Read the model definition and answer for the solid it produces. Units are mm, in the model's axes. A direction names the side the tool comes from. Coordinates: 2 decimals unless noted, no trailing zeros. Write each loop counter-clockwise with the first axis right and the second up, starting at its lowest first coordinate (ties: lowest second). Pieces come first, ordered by that corner, then holes. Notation, with made-up numbers: (24, 15) -> (60, 15) arc R27 cw to (60, 36) -> close; hole circle Ø1 at (47, 2.5). An arc over 180 degrees is marked (long way). Return JSON: item names as keys, results as strings.
from build123d import *

# Parameters (mm, degrees)
SKETCH1_W           = 60.325
SKETCH1_H           = 21.59
REVOLVE2_ANGLE      = 19
CIRPATTERN2_COUNT   = 4
BOSS_EXTRUDE1_DEPTH = 4.7625
SKETCH8_R           = 3.175


with BuildPart() as part:
    # Sketch1 → Revolve1 (revolve)
    with BuildSketch(Plane.XY, mode=Mode.PRIVATE) as revolve1_sk:
        with Locations((30.1625, 10.795)):
            Rectangle(SKETCH1_W, SKETCH1_H)
    revolve(revolve1_sk.sketch.rotate(Axis((0, 0, 0), (0, 1, 0)), 90), axis=Axis((0, 0, 0), (0, 1, 0)))

    # Sketch4 → Revolve2 (revolve)
    with BuildSketch(Plane.XY):
        with BuildLine():
            Line((60.325, 0), (60.325, 6.35))
            Line((60.325, 6.35), (58.7375, 6.35))
            Line((58.7375, 6.35), (58.7375, 0))
            ThreePointArc((58.7375, 0), (53.750434196, -14.582118625), (40.878125, -23.056353983))
            ThreePointArc((40.878125, -23.056353983), (12.559044769, -41.69967177), (1.5875, -73.780332745))
            Line((1.5875, -73.780332745), (1.5875, -76.2))
            Line((1.5875, -76.2), (3.175, -76.2))
            Line((3.175, -76.2), (3.175, -73.780332745))
            ThreePointArc((3.175, -73.780332745), (13.814073716, -42.671813012), (41.275, -24.593444248))
            ThreePointArc((41.275, -24.593444248), (55.005463142, -15.554259867), (60.325, 0))
        make_face()
    revolve2 = revolve(axis=Axis((0, 0, 0), (0, -1, 0)), revolution_arc=REVOLVE2_ANGLE)

    # CirPattern2: Revolve2 ×4 about axis
    cirpattern2_axis = Axis((0, 0, 0), (0, 1, 0))
    for i in range(1, CIRPATTERN2_COUNT):
        add(revolve2.rotate(cirpattern2_axis, i * 360 / CIRPATTERN2_COUNT))

    # Sketch6 → Boss-Extrude1 (add, symmetric)
    with BuildSketch(Plane.XY):
        with BuildLine():
            Line((3.175, -76.2), (3.175, -76.99375))
            ThreePointArc((3.175, -76.99375), (3.746845437, -79.881464155), (5.376067541, -82.333307459))
            ThreePointArc((5.376067541, -82.333307459), (0, -95.25), (-5.376067541, -82.333307459))
            ThreePointArc((-5.376067541, -82.333307459), (-3.746845437, -79.881464155), (-3.175, -76.99375))
            Line((-3.175, -76.99375), (-3.175, -76.2))
            Line((-3.175, -76.2), (-1.5875, -76.2))
            Line((-1.5875, -76.2), (-1.5875, -76.99375))
            ThreePointArc((-1.5875, -76.99375), (-2.279153864, -80.486474647), (-4.249717393, -83.45200831))
            ThreePointArc((-4.249717393, -83.45200831), (0, -93.6625), (4.249717393, -83.45200831))
            ThreePointArc((4.249717393, -83.45200831), (2.279153864, -80.486474647), (1.5875, -76.99375))
            Line((1.5875, -76.99375), (1.5875, -76.2))
            Line((1.5875, -76.2), (3.175, -76.2))
        make_face()
    extrude(amount=BOSS_EXTRUDE1_DEPTH, both=True)

    # Sweep1: sweep along a path in Sketch7
    with BuildLine(Plane.XY) as sweep1_path:
        Line((6.35, 21.59), (6.35, 27.94))
        ThreePointArc((6.35, 27.94), (0, 34.29), (-6.35, 27.94))
        Line((-6.35, 27.94), (-6.35, 21.59))
    # Sketch8 → Sweep1 (sweep)
    with BuildSketch(Plane(origin=(0, 21.59, 0), x_dir=(1, 0, 0), z_dir=(0, 1, 0))):
        with Locations((6.35, 0)):
            Circle(SKETCH8_R)
    sweep(path=sweep1_path.line)


solid = part.part
1. For a pull along X with two mould halves and no side action, classify faces 4 (the face through (-5, -84, 4.762)), 5 (the face through (2.298, -80.533, 0.067)), 6 (the face through (-9.325, -29.456, 27.083)) as +X half, -X half, draft (parallel to the pull), parting line (faces both ways), or undercut.
Taken from the geometry:
{"face 4": "draft", "face 5": "undercut", "face 6": "-X half"}
2. The part is cut by section A-A (y = -64.5). Determine the outline of the cut face in (x, z), then the cut area to 3 significant figures.
Taken from the geometry:
{"outline": "(-4.03, 0) arc R4.03 ccw to (-3.81, -1.31) -> (-2.28, -0.79) arc R2.42 cw to (-2.42, 0) -> close; (-1.31, 3.81) -> (-0.79, 2.28) arc R2.42 cw to (0, 2.42) -> (0, 4.03) arc R4.03 ccw to start; (0, -4.03) arc R4.03 ccw to (1.31, -3.81) -> (0.79, -2.28) arc R2.42 cw to (0, -2.42) -> close; (2.28, 0.79) arc R2.42 cw to (2.42, 0) -> (4.03, 0) arc R4.03 ccw to (3.81, 1.31) -> close", "area": "6.90 mm2"}
3. The part is cut by section B-B (y = 25.5). Determine the outline of the cut face in (x, z) (3 decimals), then the cut area to 3 significant figures.
Taken from the geometry:
{"outline": "circle Ø6.35 at (-6.35, 0); circle Ø6.35 at (6.35, 0)", "area": "63.3 mm2"}
4. Consider L1, parallel to Y at x = 0, z = 1; L2, parallel to Y at x = 13, z = 32; L3, parallel to Y at x = 53, z = 5. Determine where each line is inside the solid, lowest interval first.
Taken from the geometry:
{"L1": "y = -95.25 to -93.66, 0 to 21.59, 31.28 to 37.3", "L2": "y = 0 to 21.59", "L3": "y = -17.6 to -15.22, 0 to 21.59"}
5. Flat-ended cylindrical pins translate along their axes: pin 1 Ø1 at (y, z) = (16, 21.5) entering from +X; pin 2 Ø0.6 at (y, z) = (-77, 1.5) entering from -X; pin 3 Ø17.5 at (x, y) = (-28.5, -20) entering from +Z. Find the tip coordinate at first contact, or state that the pin passes through.
Taken from the geometry:
{"pin 1": "stops at x = 56.55", "pin 2": "stops at x = -3.18", "pin 3": "stops at z = 0"}
6. A tool of negligible diameter and unlimited length cuts with its end or side. For faces 1 (the face through (9.325, -29.456, -27.083)), 2 (the face through (27.083, -29.456, 9.325)), 3 (the face through (29, -29, 0)), from which of +Z, -Z, +X, -X, +Y, -Y can it reach the whole face along a straight path? Write none if from no direction.
Taken from the geometry:
{"face 1": "+Z, +X", "face 2": "+Z, -X", "face 3": "-Z, +X"}
